Verification items for the finished model (mm, model axes). Face numbers are marked on the shaded views. A direction names the side the tool comes from. Give positions to 0.01 mm unless a question says otherwise; leave off trailing zeros. Loops run counter-clockwise (first coordinate to the right, second up) from the corner with the lowest first, then second, coordinate; pieces in that order, holes last. Notation, with made-up numbers: (19, -20) - (70, -20) arc R14 cw to (70, -6) - close; hole circle Ø5 at (61.5, -10.5). An arc over 180 degrees is marked (long way). One line per question, with ' | ' between items. Start each with the question number.
1. Depth check by flat-ended pin: pin 1 Ø1 at (x, y) = (25.5, 62.5) entering from +Z; pin 2 Ø5 at (x, z) = (-19, -44) entering from +Y; pin 3 Ø19.5 at (y, z) = (62.5, -34.5) entering from +X; pin 4 Ø24 at (x, z) = (25, -35) entering from +Y. Enter the tip coordinate at first touch or a pass-through.
2. Mould release check, pull along Z, two halves, no side actions. Record for the marked faces 5, 6 and 7: +Z half, -Z half, draft (parallel to the pull), parting line (faces both ways), or undercut.
3. Tool access check on the marked faces 1, 2, 3 and 4. Record the directions out of +Z, -Z, +X, -X, +Y, -Y that give a thin tool (end or side, any length) a straight path to the whole face; none if there is none.
4. Section check C-C, the plane y = 30.5. Enter the section's corners in (x, z), then the cut area to 3 significant figures.
5. Section check D-D, the plane x = -52.5. Enter the section's corners in (y, z), then the cut area to 3 significant figures.
6. Thickness scan on line 1 along Z through (x, y) = (25, 43); line 2 along X through (y, z) = (28.5, -8); line 3 along X through (y, z) = (80, -11.5). Record the ranges inside material, lowest first. Write a range as from..to.
7. Section check A-A, the plane z = -58. Enter the section's corners in (x, y).
8. Section check B-B, the plane x = 14.5. Enter the section's corners in (y, z).
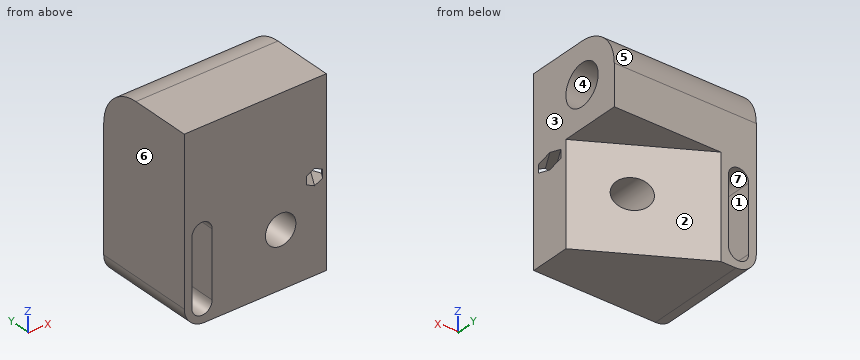
from build123d import *

# Parameters (mm, degrees)
SKETCH1_R           = 15
BOSS_EXTRUDE1_DEPTH = 100
CUT_EXTRUDE1_DEPTH  = 100
FILLET1_R           = 40
SKETCH3_R           = 20
CUT_EXTRUDE2_DEPTH  = 105
CUT_EXTRUDE3_DEPTH  = 191.523897853


with BuildPart() as part:
    # Sketch1 → Boss-Extrude1 (new body)
    with BuildSketch(Plane(origin=(0, 0, 0), x_dir=(1, 0, 0), z_dir=(0, 1, 0))):
        with BuildLine():
            Line((-50, -90), (70, -90))
            Line((70, -90), (70, 90))
            Line((70, 90), (-70, 90))
            Line((-70, 90), (-70, -70))
            ThreePointArc((-70, -70), (-64.142135624, -84.142135624), (-50, -90))
        make_face()
        with Locations(Location((25, -35, 0), (0, 0, 270))):
            Circle(SKETCH1_R, mode=Mode.SUBTRACT)
        with BuildLine():
            Line((-42.5, -7.5), (-42.5, -72.5))
            ThreePointArc((-42.5, -72.5), (-52.5, -82.5), (-62.5, -72.5))
            Line((-62.5, -72.5), (-62.5, -7.5))
            ThreePointArc((-62.5, -7.5), (-52.5, 2.5), (-42.5, -7.5))
        make_face(mode=Mode.SUBTRACT)
    extrude(amount=BOSS_EXTRUDE1_DEPTH)

    # Sketch2 → Cut-Extrude1 (cut)
    with BuildSketch(Plane.XY.offset(90)):
        Polygon((-35, 100), (70, 40), (70, 100), align=None)
    extrude(amount=-CUT_EXTRUDE1_DEPTH, mode=Mode.SUBTRACT)

    # Fillet1
    fillet1_edges = [part.edges().sort_by_distance(p)[0] for p in [
        (0, 100, -90),
    ]]
    fillet(fillet1_edges, radius=FILLET1_R)

    # Sketch3 → Cut-Extrude2 (cut)
    with BuildSketch(Plane(origin=(70, 0, 0), x_dir=(0, 0, -1), z_dir=(1, 0, 0))):
        with Locations((50, 60)):
            Circle(SKETCH3_R)
    extrude(amount=-CUT_EXTRUDE2_DEPTH, mode=Mode.SUBTRACT)

    # Sketch6 → Cut-Extrude3 (cut, through all)
    with BuildSketch(Plane(origin=(60.801270189, 105.310889132, 0), x_dir=(0, 0, -1), z_dir=(0.499999999999998, 0.8660254037844398, 0))):
        Polygon((8, -50.621778265), (4, -43.693575035), (-4, -43.693575035), (-8, -50.621778265), (-4, -57.549981495), (4, -57.549981495), align=None)
    extrude(amount=-CUT_EXTRUDE3_DEPTH, mode=Mode.SUBTRACT)


with BuildPart() as body_2:
    # Mirror1: mirrored copy
    add(part.part.mirror(Plane(origin=(-50, 100, 90), x_dir=(1, 0, 0), z_dir=(0, 0, -1))))


with BuildPart() as body_2_1:
    # Body-Move/Copy2: moved
    add(body_2.part.moved(Location((0, 0, -180))))


solid = body_2_1.part
Results list:
1) pin 1: z = 89.95 | pin 2: y = 92.29 | pin 3: x = 47.69 | pin 4: through
2) face 5: +Z half | face 6: draft | face 7: undercut
3) face 1: +Y, -Y | face 2: -Z, +X, +Y | face 3: +Z, -Z, +X, +Y, -Y | face 4: +X
4) outline: (-70, -70) arc R20 ccw to (-50, -90) - (70, -90) - (70, -4.97) - (68.06, -4) - (68.06, 4) - (70, 4.97) - (70, 90) - (-70, 90) - close; hole (-62.5, -72.5) arc R10 ccw to (-42.5, -72.5) - (-42.5, -7.5) arc R10 ccw to (-62.5, -7.5) - close; hole circle Ø30 at (25, -35) | area: 22,800 mm²
5) outline: (0, -89.84) - (100, -89.84) - (100, -82.5) - (0, -82.5) - close; (0, 2.5) - (100, 2.5) - (100, 50) arc R40 ccw to (60, 90) - (0, 90) - close | area: 9,140 mm²
6) line 1: -90..-50, -20..39.46, 60.54..90 | line 2: -70..-62.5, -42.5..70 | line 3: -70..-62.5, -42.5..0
7) outline: (-70, 0) - (-62.5, 0) - (-62.5, 100) - (-70, 100) - close; (-42.5, 0) - (70, 0) - (70, 40) - (-35, 100) - (-42.5, 100) - close
8) outline: (0, -90) - (71.71, -90) - (71.71, -45.71) - (0, -45.71) - close; (0, -24.29) - (71.71, -24.29) - (71.71, 10) - (100, 10) - (100, 50) arc R40 ccw to (60, 90) - (0, 90) - close; hole circle Ø40 at (60, 50)
